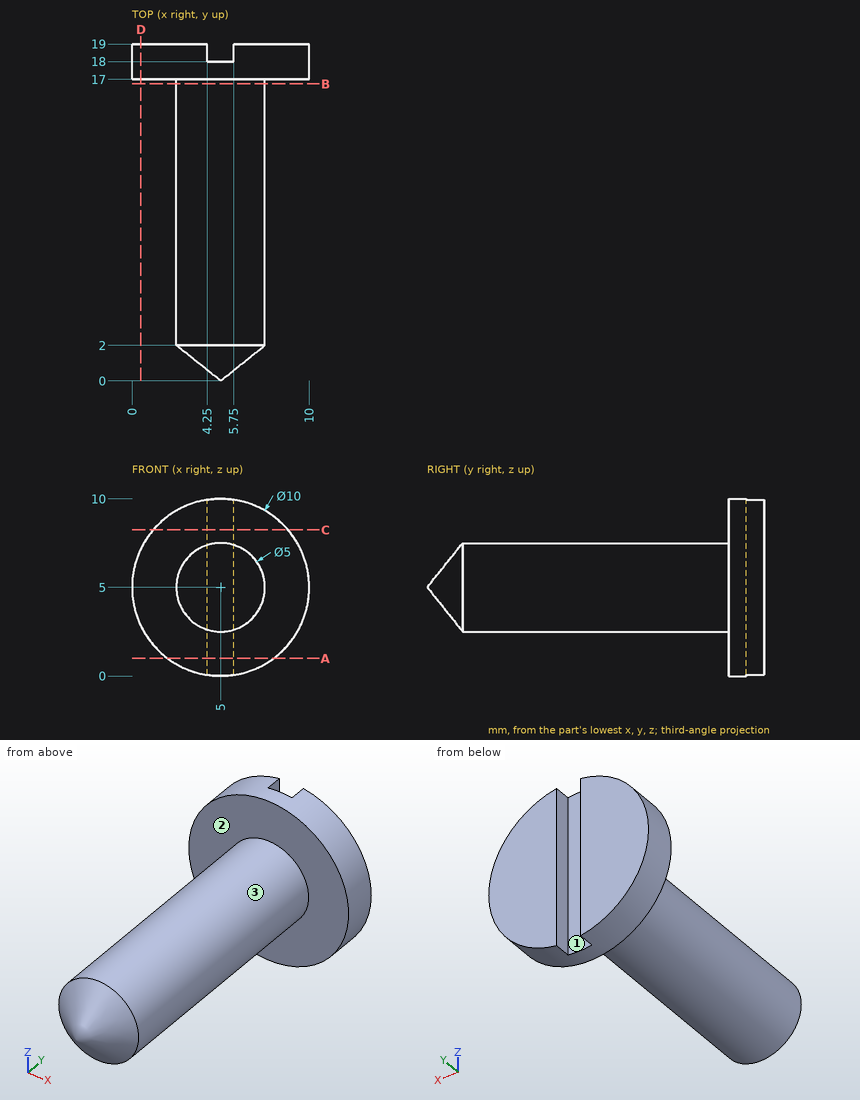
Geometry check sheet. Reference: drawing and pictorial views, mm from the part's lowest x, y, z. Coordinates: 2 decimals unless noted, no trailing zeros. Order: outer loops, then holes, each group sorted by start corner. A loop starts at its lowest first (then second) coordinate and runs counter-clockwise, first axis right, second up. Notation, with made-up numbers: (77, -12.5) -> (87, -12.5) arc R16 cw to (87, -6.5) -> close; hole circle Ø6 at (60.25, 39.5). An arc over 180 degrees is marked (long way). Put each result on its own line as item: value. Start each with the question number.
1) Cross-section at D-D (x = 0.5). Enter the section's corners in (y, z).
2) Cross-section at C-C (z = 8.25). Enter the section's corners in (x, y).
3) Release check for a two-part mould opening along X. For the marked faces 1, 2 and 3 record: pulls with the +X half, pulls with the -X half, needs draft (parallel to the pull), parting line crosses it, or undercut.
4) Go/stop test with flat-tipped pins: pin 1 (1 mm diameter, centred on x = 4, y = 14, fed in from +Z); pin 2 (6 mm diameter, centred on x = 6.5, y = 8.5, fed in from +Z); pin 3 (0.5 mm diameter, centred on y = 18.5, z = 5.5, fed in from -X); pin 4 (1 mm diameter, centred on y = 2, z = 8.5, fed in from -X). Record where each tip stops, or that it passes through.
5) Material ranges on L1, parallel to Y at x = 0.75, z = 3.25; L2, parallel to Z at x = 5.5, y = 4.75; L3, parallel to Z at x = 3, y = 6.5, recorded low to high.
6) Cross-section at A-A (z = 1). Enter the section's corners in (x, y).
7) Cross-section at B-B (y = 16.75). Enter the section's corners in (x, z), plus the area to 3 significant figures.
Geometry check:
1. outline: (17, 2.82) -> (19, 2.82) -> (19, 7.18) -> (17, 7.18) -> close
2. outline: (1.2, 17) -> (8.8, 17) -> (8.8, 19) -> (5.75, 19) -> (5.75, 18) -> (4.25, 18) -> (4.25, 19) -> (1.2, 19) -> close
3. face 1: undercut
3. face 2: needs draft
3. face 3: parting line crosses it
4. pin 1: stops at z = 7.45
4. pin 2: stops at z = 7.5
4. pin 3: stops at x = 0.01
4. pin 4: passes through
5. L1: y = 17 to 19
5. L2: z = 2.55 to 7.45
5. L3: z = 3.5 to 6.5
6. outline: (2, 17) -> (8, 17) -> (8, 19) -> (5.75, 19) -> (5.75, 18) -> (4.25, 18) -> (4.25, 19) -> (2, 19) -> close
7. outline: circle Ø5 at (5, 5)
7. area: 19.6 mm^2
